```python
from build123d import *

# Parameters (mm, degrees)
SKETCH_1_W          = 180
SKETCH_1_H          = 55
SKETCH_1_W_2        = 176
SKETCH_1_H_2        = 51
EXTRUDE_1_DEPTH     = 10
SKETCH_4_W          = 180
SKETCH_4_H          = 55
EXTRUDE_2_DEPTH     = 2.5
SKETCH_5_W          = 10.5
SKETCH_5_H          = 5.5
CUT_EXTRUDE_1_DEPTH = 2.5
SKETCH_7_R          = 3
EXTRUDE_3_DEPTH     = 12
SKETCH_8_R          = 1.517316024
SKETCH_8_R_2        = 1.4341078
CUT_EXTRUDE_2_DEPTH = 8
SKETCH_9_R          = 5.5
CUT_EXTRUDE_3_DEPTH = 8
SKETCH_10_R         = 1.75
CUT_EXTRUDE_4_DEPTH = 8
SKETCH_12_W         = 2
SKETCH_12_H         = 24.5
CUT_EXTRUDE_5_DEPTH = 8
SKETCH_13_R         = 5.4
CUT_EXTRUDE_6_DEPTH = 8
SKETCH_15_W         = 50
SKETCH_15_H         = 29
CUT_EXTRUDE_7_DEPTH = 8
SKETCH_16_W         = 54
SKETCH_16_H         = 33
SKETCH_16_W_2       = 50
SKETCH_16_H_2       = 29
EXTRUDE_2_2_DEPTH   = 2
CHAMFER_1_SIZE      = 2
CHAMFER_2_SIZE      = 1
CHAMFER_3_SIZE      = 1
CHAMFER_4_SIZE      = 1
CHAMFER_5_SIZE      = 1
FILLET_1_R          = 2


with BuildPart() as part:
    # Эскиз1 → Вытянуть-Тонкостенный1 (new body)
    with BuildSketch(Plane.XY):
        Rectangle(SKETCH_1_W, SKETCH_1_H)
        Rectangle(SKETCH_1_W_2, SKETCH_1_H_2, mode=Mode.SUBTRACT)
    extrude(amount=EXTRUDE_1_DEPTH)

    # Эскиз4 → Extrude 2 (add)
    with BuildSketch(Plane(origin=(0, 0, 0), x_dir=(-1, 0, 0), z_dir=(0, 0, -1))):
        Rectangle(SKETCH_4_W, SKETCH_4_H)
    extrude(amount=EXTRUDE_2_DEPTH)

    # Эскиз5 → Вырез-Вытянуть1 (cut)
    with BuildSketch(Plane(origin=(0, 0, -2.5), x_dir=(-1, 0, 0), z_dir=(0, 0, -1))):
        with Locations((60, 15.5)):
            Rectangle(SKETCH_5_W, SKETCH_5_H)
    extrude(amount=-CUT_EXTRUDE_1_DEPTH, mode=Mode.SUBTRACT)

    # Эскиз7 → Бобышка-Вытянуть3 (add)
    with BuildSketch(Plane.XY):
        with Locations(Location((-51, 15.5, 0), (0, 0, 180))):
            Circle(SKETCH_7_R)
        with Locations(Location((-69, 15.5, 0), (0, 0, 180))):
            Circle(SKETCH_7_R)
    extrude(amount=EXTRUDE_3_DEPTH)

    # Эскиз8 → Вырез-Вытянуть2 (cut)
    with BuildSketch(Plane.XY.offset(12)):
        with Locations((-69, 15.5)):
            Circle(SKETCH_8_R)
        with Locations((-51, 15.5)):
            Circle(SKETCH_8_R_2)
    extrude(amount=-CUT_EXTRUDE_2_DEPTH, mode=Mode.SUBTRACT)

    # Эскиз9 → Вырез-Вытянуть3 (cut)
    with BuildSketch(Plane(origin=(0, 0, -2.5), x_dir=(-1, 0, 0), z_dir=(0, 0, -1))):
        with Locations((60, -10.5)):
            Circle(SKETCH_9_R)
    extrude(amount=-CUT_EXTRUDE_3_DEPTH, mode=Mode.SUBTRACT)

    # Эскиз10 → Вырез-Вытянуть4 (cut)
    with BuildSketch(Plane(origin=(0, 0, -2.5), x_dir=(-1, 0, 0), z_dir=(0, 0, -1))):
        with Locations((25, 14)):
            Circle(SKETCH_10_R)
        with Locations((25, -14)):
            Circle(SKETCH_10_R)
    extrude(amount=-CUT_EXTRUDE_4_DEPTH, mode=Mode.SUBTRACT)

    # Эскиз12 → Вырез-Вытянуть5 (cut)
    with BuildSketch(Plane(origin=(0, 0, -2.5), x_dir=(-1, 0, 0), z_dir=(0, 0, -1))):
        with Locations((29, 0)):
            Rectangle(SKETCH_12_W, SKETCH_12_H)
    extrude(amount=-CUT_EXTRUDE_5_DEPTH, mode=Mode.SUBTRACT)

    # Эскиз13 → Вырез-Вытянуть6 (cut)
    with BuildSketch(Plane(origin=(0, 0, -2.5), x_dir=(-1, 0, 0), z_dir=(0, 0, -1))):
        with Locations((-4, 0)):
            Circle(SKETCH_13_R)
    extrude(amount=-CUT_EXTRUDE_6_DEPTH, mode=Mode.SUBTRACT)

    # Эскиз15 → Вырез-Вытянуть7 (cut)
    with BuildSketch(Plane(origin=(0, 0, -2.5), x_dir=(-1, 0, 0), z_dir=(0, 0, -1))):
        with Locations((-55, 0)):
            Rectangle(SKETCH_15_W, SKETCH_15_H)
    extrude(amount=-CUT_EXTRUDE_7_DEPTH, mode=Mode.SUBTRACT)

    # Эскиз16 → Extrude 2 2 (add)
    with BuildSketch(Plane.XY):
        with Locations((55, 0)):
            Rectangle(SKETCH_16_W, SKETCH_16_H)
        with Locations((55, 0)):
            Rectangle(SKETCH_16_W_2, SKETCH_16_H_2, mode=Mode.SUBTRACT)
    extrude(amount=EXTRUDE_2_2_DEPTH)

    # Фаска1
    chamfer_1_edges = [part.edges().sort_by_distance(p)[0] for p in [
        (80, 0, -2.5),
        (55, -14.5, -2.5),
        (30, 0, -2.5),
        (55, 14.5, -2.5),
    ]]
    chamfer(chamfer_1_edges, length=CHAMFER_1_SIZE)

    # Фаска2
    chamfer_2_edges = [part.edges().sort_by_distance(p)[0] for p in [
        (-30, 0, -2.5),
        (-29, 12.25, -2.5),
        (-28, 0, -2.5),
        (-29, -12.25, -2.5),
    ]]
    chamfer(chamfer_2_edges, length=CHAMFER_2_SIZE)

    # Фаска3
    chamfer_3_edges = [part.edges().sort_by_distance(p)[0] for p in [
        (-65.25, 15.5, -2.5),
        (-60, 18.25, -2.5),
        (-54.75, 15.5, -2.5),
        (-60, 12.75, -2.5),
    ]]
    chamfer(chamfer_3_edges, length=CHAMFER_3_SIZE)

    # Фаска4
    # the kernel refuses this chamfer: 1 mm, written as the material it adds along each edge
    with BuildSketch(Plane(origin=(-51, 15.5, 0), x_dir=(-1, 0, 0), z_dir=(0, 1, 0))) as chamfer_4_piece_1_section:
        Polygon((3 + CHAMFER_4_SIZE, 0), (3, CHAMFER_4_SIZE), (3, 0), align=None)
    chamfer_4_piece_1 = revolve(axis=Axis((-51, 15.5, 0), (0, 0, 1)), mode=Mode.PRIVATE)
    chamfer_4_piece_1 = split(chamfer_4_piece_1, bisect_by=Plane(origin=(-54.75, 15.5, 0.484065112), z_dir=(1, 0, 0)), keep=Keep.TOP, mode=Mode.PRIVATE)
    add(chamfer_4_piece_1)
    with BuildSketch(Plane(origin=(-69, 15.5, 0), x_dir=(-1, 0, 0), z_dir=(0, 1, 0))) as chamfer_4_piece_2_section:
        Polygon((3 + CHAMFER_4_SIZE, 0), (3, CHAMFER_4_SIZE), (3, 0), align=None)
    chamfer_4_piece_2 = revolve(axis=Axis((-69, 15.5, 0), (0, 0, 1)), mode=Mode.PRIVATE)
    chamfer_4_piece_2 = split(chamfer_4_piece_2, bisect_by=Plane(origin=(-65.25, 15.5, 0.484065116), z_dir=(-1, 0, 0)), keep=Keep.TOP, mode=Mode.PRIVATE)
    add(chamfer_4_piece_2)

    # Фаска5
    chamfer_5_edges = [part.edges().sort_by_distance(p)[0] for p in [
        (88, 0, 0),
        (0, 25.5, 0),
        (-88, 0, 0),
        (0, -25.5, 0),
    ]]
    chamfer(chamfer_5_edges, length=CHAMFER_5_SIZE)

    # Скругление1
    fillet_1_edges = [part.edges().sort_by_distance(p)[0] for p in [
        (-90, 0, -2.5),
        (0, 27.5, -2.5),
        (90, 0, -2.5),
        (0, -27.5, -2.5),
    ]]
    fillet(fillet_1_edges, radius=FILLET_1_R)


solid = part.part
```
The listing builds one solid part. Answer for the finished solid, in the listing's coordinates (mm). A direction names the side the tool comes from. Give positions to 0.01 mm unless a question says otherwise; leave off trailing zeros. Order: outer loops, then holes, each group sorted by start corner. A loop starts at its lowest first (then second) coordinate and runs counter-clockwise, first axis right, second up. Notation, with made-up numbers: (-24.75, 64) -> (0.25, 64) arc R27 cw to (0.25, 96) -> close; hole circle Ø10 at (65, -7). An arc over 180 degrees is marked (long way). Answer as a JSON object with one key per item and string values. Group by question number.
Item 1: The part is cut by section D-D on x = -60. Write down the section's boundary in (y, z), and give its area (3 significant figures).
Item 2: A tool of negligible diameter and unlimited length cuts with its end or side. For faces 4 (the flat face through (-18, 0, -2.5)), 5 (the flat face through (53, -15, 2)), from which of +Z, -Z, +X, -X, +Y, -Y can it reach the whole face along a straight path? Write none if from no direction.
Item 3: The part is cut by section A-A on z = 7.25. Write down the section's boundary in (x, y).
Item 4: Determine the mould class of faces 1 (the flat face through (-90, 0, 5)), 2 (the flat face through (-52, 17, 12)), 3 (the flat face through (88, 0, 5)) for opening direction X: pulls with the +X half, pulls with the -X half, needs draft (parallel to the pull), parting line crosses it, or undercut.
Item 5: Flat-ended cylindrical pins translate along their axes: pin 1 (1.2 mm diameter, centred on x = -29, z = -1, fed in from -Y); pin 2 (0.8 mm diameter, centred on y = -2, z = -1, fed in from -X). Find the tip coordinate at first contact, or state that the pin passes through.
Item 6: The part is cut by section B-B on x = -25. Write down the section's boundary in (y, z).
Item 7: The part is cut by section C-C on x = 4. Write down the section's boundary in (y, z), and give its area (3 significant figures).
Item 8: Consider L1, parallel to Y at x = 4, z = 3; L2, parallel to X at y = 15.5, z = 1.5; L3, parallel to X at y = -15, z = 8.5. Determine where each line is inside the solid, lowest interval first. Write a range as from..to.
Result set:
{
 "1": {"outline": "(-27.5, -0.5) arc R2 ccw to (-25.5, -2.5) -> (-16, -2.5) -> (-16, 0) -> (-24.5, 0) -> (-25.5, 1) -> (-25.5, 10) -> (-27.5, 10) -> close; (-5, -2.5) -> (11.75, -2.5) -> (12.75, -1.5) -> (12.75, 0) -> (-5, 0) -> close; (18.25, -1.5) -> (19.25, -2.5) -> (25.5, -2.5) arc R2 ccw to (27.5, -0.5) -> (27.5, 10) -> (25.5, 10) -> (25.5, 1) -> (24.5, 0) -> (18.25, 0) -> close", "area": "135 mm²"},
 "2": {"face 4": "-Z, +X, -X, +Y, -Y", "face 5": "+Z"},
 "3": {"outline": "(-90, -27.5) -> (90, -27.5) -> (90, 27.5) -> (-90, 27.5) -> close; circle Ø6 at (-69, 15.5); circle Ø6 at (-51, 15.5); hole (-88, -25.5) -> (88, -25.5) -> (88, 25.5) -> (-88, 25.5) -> close; hole circle Ø3.03 at (-69, 15.5); hole circle Ø2.87 at (-51, 15.5)"},
 "4": {"face 1": "pulls with the -X half", "face 2": "needs draft", "face 3": "undercut"},
 "5": {"pin 1": "y = -27.5", "pin 2": "x = -90"},
 "6": {"outline": "(-27.5, -0.5) arc R2 ccw to (-25.5, -2.5) -> (-15.75, -2.5) -> (-15.75, 0) -> (-24.5, 0) -> (-25.5, 1) -> (-25.5, 10) -> (-27.5, 10) -> close; (-12.25, -2.5) -> (12.25, -2.5) -> (12.25, 0) -> (-12.25, 0) -> close; (15.75, -2.5) -> (25.5, -2.5) arc R2 ccw to (27.5, -0.5) -> (27.5, 10) -> (25.5, 10) -> (25.5, 1) -> (24.5, 0) -> (15.75, 0) -> close"},
 "7": {"outline": "(-27.5, -0.5) arc R2 ccw to (-25.5, -2.5) -> (-5.4, -2.5) -> (-5.4, 0) -> (-24.5, 0) -> (-25.5, 1) -> (-25.5, 10) -> (-27.5, 10) -> close; (5.4, -2.5) -> (25.5, -2.5) arc R2 ccw to (27.5, -0.5) -> (27.5, 10) -> (25.5, 10) -> (25.5, 1) -> (24.5, 0) -> (5.4, 0) -> close", "area": "150 mm²"},
 "8": {"L1": "-27.5..-25.5, 25.5..27.5", "L2": "-90..-88, -72..-66, -54..-48, 28..82, 88..90", "L3": "-90..-88, 88..90"}
}
